```python
from build123d import *

# Parameters (mm, degrees)
F0_R     = 1.2
F0_R_2   = 1.5
F1_DEPTH = 0.744
F2_W     = 0.744
F2_H     = 103
F2_H_2   = 102.999995
F3_DEPTH = 8
F4_R     = 1


# Not quite as in the source:
# - ends of sketch curves that miss each other by under 0.0002 mm in the source are joined


with BuildPart() as f1:
    # F0 (on Top) → F1 (new body)
    with BuildSketch(Plane.XY):
        with BuildLine():
            Line((-39.500012, -54.499996), (30.29995, -54.500001))
            Line((30.29995, -54.500001), (30.29995, 52.4999855731))
            ThreePointArc((30.29995, 52.4999855731), (29.714163765, 53.9141989328), (28.2999505731, 54.4999855731))
            Line((28.2999505731, 54.4999855731), (-37.5000114269, 54.5000044269))
            ThreePointArc((-37.5000114269, 54.5000044269), (-38.9142253598, 53.9142181919), (-39.500012, 52.5000044269))
            Line((-39.500012, 52.5000044269), (-39.500012, -54.499996))
        make_face()
        with Locations((-23.649861, -42.950105)):
            Circle(F0_R, mode=Mode.SUBTRACT)
        with Locations((-27.501189, -24.642994)):
            Circle(F0_R_2, mode=Mode.SUBTRACT)
        with BuildLine():
            Line((-20.749991, -8.499996), (-24.749991, -8.499996))
            ThreePointArc((-24.749991, -8.499996), (-25.2803207323, -8.2803268537), (-25.499992, -7.749998))
            Line((-25.499992, -7.749998), (-25.499992, -4.749996))
            ThreePointArc((-25.499992, -4.749996), (-25.2803225001, -4.2196659141), (-24.749993, -3.999995))
            Line((-24.749993, -3.999995), (-20.749991, -3.999995))
            ThreePointArc((-20.749991, -3.999995), (-20.2196642677, -4.2196641463), (-19.999993, -4.749993))
            Line((-19.999993, -4.749993), (-19.999993, -7.749995))
            ThreePointArc((-19.999993, -7.749995), (-20.2196621463, -8.2803247323), (-20.749991, -8.499996))
        make_face(mode=Mode.SUBTRACT)
        with Locations((14.450063, -42.950105)):
            Circle(F0_R, mode=Mode.SUBTRACT)
        with Locations((-1.248788, -22.556994)):
            Circle(F0_R_2, mode=Mode.SUBTRACT)
        with Locations((8.00001, -14.749994)):
            Circle(F0_R_2, mode=Mode.SUBTRACT)
        with BuildLine():
            ThreePointArc((2.500013, -6.999991), (1.9696832677, -6.7803218537), (1.750012, -6.249993))
            Line((1.750012, -6.249993), (1.750012, -2.249993))
            ThreePointArc((1.750012, -2.249993), (1.9696814999, -1.7196629141), (2.500011, -1.499992))
            Line((2.500011, -1.499992), (5.500012, -1.499992))
            ThreePointArc((5.500012, -1.499992), (6.0303420859, -1.7196614999), (6.250013, -2.249991))
            Line((6.250013, -2.249991), (6.250013, -6.249993))
            ThreePointArc((6.250013, -6.249993), (6.0303438537, -6.7803197323), (5.500015, -6.999991))
            Line((5.500015, -6.999991), (2.500013, -6.999991))
        make_face(mode=Mode.SUBTRACT)
        with BuildLine():
            ThreePointArc((17.750011, -4.249994), (17.9696801463, -3.7196642677), (18.500009, -3.499993))
            Line((18.500009, -3.499993), (22.500011, -3.499993))
            ThreePointArc((22.500011, -3.499993), (23.0303390859, -3.7196624999), (23.25001, -4.249992))
            Line((23.25001, -4.249992), (23.25001, -7.249993))
            ThreePointArc((23.25001, -7.249993), (23.0303405001, -7.7803230859), (22.500011, -7.999994))
            Line((22.500011, -7.999994), (18.500012, -7.999995))
            ThreePointArc((18.500012, -7.999995), (17.9696822677, -7.7803248537), (17.750011, -7.249996))
            Line((17.750011, -7.249996), (17.750011, -4.249994))
        make_face(mode=Mode.SUBTRACT)
        with BuildLine():
            Line((-13.749987, 17.000004), (-13.749987, 12.500005))
            ThreePointArc((-13.749987, 12.500005), (-13.9696564999, 11.9696749141), (-14.499986, 11.750004))
            Line((-14.499986, 11.750004), (-26.749989, 11.750004))
            ThreePointArc((-26.749989, 11.750004), (-27.2803170859, 11.9696734999), (-27.499988, 12.500003))
            Line((-27.499988, 12.500003), (-27.499988, 17.000004))
            ThreePointArc((-27.499988, 17.000004), (-27.2803185001, 17.5303340859), (-26.749989, 17.750005))
            Line((-26.749989, 17.750005), (-14.499988, 17.750005))
            ThreePointArc((-14.499988, 17.750005), (-13.9696579141, 17.5303355001), (-13.749987, 17.000004))
        make_face(mode=Mode.SUBTRACT)
        with Locations((-14.999987, 26.750007)):
            Circle(F0_R_2, mode=Mode.SUBTRACT)
        with Locations((-6.249987, 26.750005)):
            Circle(F0_R_2, mode=Mode.SUBTRACT)
        with Locations((-36.499988, 51.750005)):
            Circle(F0_R, mode=Mode.SUBTRACT)
        with BuildLine():
            ThreePointArc((-16.999976, 30.499992), (-17.5303057323, 30.7196611463), (-17.749977, 31.24999))
            Line((-17.749977, 31.24999), (-17.749987, 41.749995))
            ThreePointArc((-17.749987, 41.749995), (-17.5303305001, 42.2803250859), (-17.000001, 42.499996))
            Line((-17.000001, 42.499996), (-8.499988, 42.500006))
            ThreePointArc((-8.499988, 42.500006), (-7.9696584999, 42.7196769141), (-7.749989, 43.250007))
            Line((-7.749989, 43.250007), (-7.749989, 45.750005))
            ThreePointArc((-7.749989, 45.750005), (-7.5303175001, 46.2803350859), (-6.999988, 46.500006))
            Line((-6.999988, 46.500006), (-4.249989, 46.500006))
            ThreePointArc((-4.249989, 46.500006), (-3.7196594999, 46.2803350859), (-3.49999, 45.750005))
            Line((-3.49999, 45.750005), (-3.499987, 43.250007))
            ThreePointArc((-3.499987, 43.250007), (-3.2803178537, 42.7196772677), (-2.749989, 42.500006))
            Line((-2.749989, 42.500006), (0.699984, 42.500006))
            ThreePointArc((0.699984, 42.500006), (1.2303137323, 42.2803368537), (1.449985, 41.750008))
            Line((1.449985, 41.750008), (1.449985, 41.250006))
            Line((1.449985, 41.250006), (1.449985, 31.24999))
            ThreePointArc((1.449985, 31.24999), (1.2303037323, 30.7196611463), (0.699974, 30.499992))
            Line((0.699974, 30.499992), (-16.999976, 30.499992))
        make_face(mode=Mode.SUBTRACT)
        with Locations((-1.499989, 26.750005)):
            Circle(F0_R_2, mode=Mode.SUBTRACT)
        with BuildLine():
            ThreePointArc((5.250013, 11.750004), (4.7196829141, 11.9696734999), (4.500012, 12.500003))
            Line((4.500012, 12.500003), (4.500012, 17.000004))
            ThreePointArc((4.500012, 17.000004), (4.7196811463, 17.5303337323), (5.25001, 17.750005))
            Line((5.25001, 17.750005), (17.500011, 17.750005))
            ThreePointArc((17.500011, 17.750005), (18.0303410859, 17.5303355001), (18.250012, 17.000006))
            Line((18.250012, 17.000006), (18.250012, 12.500005))
            ThreePointArc((18.250012, 12.500005), (18.0303428537, 11.9696752677), (17.500014, 11.750004))
            Line((17.500014, 11.750004), (5.250013, 11.750004))
        make_face(mode=Mode.SUBTRACT)
        with Locations((27.250012, 51.750005)):
            Circle(F0_R, mode=Mode.SUBTRACT)
    extrude(amount=F1_DEPTH)

    # F2 (on face) → F3 (join)
    with BuildSketch(Plane(origin=(0, 0, 0), x_dir=(1, 0, 0), z_dir=(0, 0, -1))):
        with Locations((29.92795, 3.000001)):
            Rectangle(F2_W, F2_H)
        with Locations((-39.128012, 2.9999985)):
            Rectangle(F2_W, F2_H_2)
    extrude(amount=-F3_DEPTH)

    # F4
    f4_edges = [f1.edges().sort_by_distance(p)[0] for p in [
        (29.92795, -54.500001, 8),
        (29.92795, 48.499999, 8),
        (-39.128012, 48.499999, 8),
        (-39.128012, -54.499996, 8),
    ]]
    fillet(f4_edges, radius=F4_R)


solid = f1.part
```
Geometry check sheet. Reference: the model listing, model coordinates, mm. A direction names the side the tool comes from. Coordinates: 2 decimals unless noted, no trailing zeros. Order: outer loops, then holes, each group sorted by start corner. A loop starts at its lowest first (then second) coordinate and runs counter-clockwise, first axis right, second up.
Q1. Tool access check on faces 1 (the face through (29.556, -2, 4)), 2 (the face through (-1.574, -24.021, 0.367)). Record the directions out of +Z, -Z, +X, -X, +Y, -Y that give a thin tool (end or side, any length) a straight path to the whole face; none if there is none.
Reply:
face 1: +Z, +Y, -Y
face 2: +Z, -Z
Q2. Sectioned sample at A-A on z = 2.75. Record the cut outline in (x, y), and give its area (3 significant figures).
Reply:
outline: (-39.5, -54.5) - (-38.76, -54.5) - (-38.76, 48.5) - (-39.5, 48.5) - close; (29.56, -54.5) - (30.3, -54.5) - (30.3, 48.5) - (29.56, 48.5) - close
area: 153 mm2
Q3. Sectioned sample at B-B on y = -17.5. Record the cut outline in (x, z).
Reply:
outline: (-39.5, 0) - (30.3, 0) - (30.3, 8) - (29.56, 8) - (29.56, 0.74) - (-38.76, 0.74) - (-38.76, 8) - (-39.5, 8) - close
Q4. Thickness scan on probe 1 along X at (y, z) = (41.5, 1.75); probe 2 along Z at (x, y) = (19.5, 44.5). Record the ranges inside material, lowest first.
Reply:
probe 1: x = -39.5 to -38.76, 29.56 to 30.3
probe 2: z = 0 to 0.74
Q5. Depth check by flat-ended pin: pin 1 Ø5 at (x, y) = (-15, 26.75) entering from +Z. Enter the tip coordinate at first touch or a pass-through.
Reply:
pin 1: stops at z = 0.74
Q6. Draft check along Y on faces 3 (the face through (-28.69, -25.56, 0.37)), 4 (the face through (-38.9, 53.93, 0.37)), 5 (the face through (-38.756, -2, 4)). Enter one of: released by +Y, released by -Y, zero draft, split by the parting line, or undercut.
Reply:
face 3: undercut
face 4: released by +Y
face 5: zero draft
